from build123d import *

# Parameters (mm, degrees)
SKETCH_W            = 104.8
SKETCH_H            = 31
PAD_DEPTH           = 1.5
HOLE_D              = 3.4
HOLE_DEPTH          = 25
HOLE_CSINK_D        = 6.1
HOLE_CSINK_ANGLE    = 90
FILLET_R            = 3.5
SKETCH002_R         = 1.8
POCKET_DEPTH        = 1.501
LINEARPATTERN_COUNT = 2
LINEARPATTERN_PITCH = 81.28


with BuildPart() as part:
    # Sketch → Pad (new body)
    with BuildSketch(Plane.XZ):
        Rectangle(SKETCH_W, SKETCH_H)
    extrude(amount=PAD_DEPTH)

    # Hole
    with Locations(Plane.XZ.offset(1.5)):
        with Locations((-48.5, 11.5), (-48.5, -11.5), (48.5, -11.5), (48.5, 11.5)):
            CounterSinkHole(HOLE_D / 2, HOLE_CSINK_D / 2, depth=HOLE_DEPTH, counter_sink_angle=HOLE_CSINK_ANGLE)

    # Fillet
    fillet_edges = [part.edges().sort_by_distance(p)[0] for p in [
        (-52.4, -0.75, 15.5),
        (52.4, -0.75, 15.5),
    ]]
    fillet(fillet_edges, radius=FILLET_R)

    # Sketch002 (on Face5 of Fillet) → Pocket (cut, through all)
    with BuildSketch(Plane.XZ.offset(1.5)):
        with Locations((-40.61, 0.03)):
            Circle(SKETCH002_R)
    pocket = extrude(amount=-POCKET_DEPTH, mode=Mode.SUBTRACT)

    # LinearPattern: Pocket ×2
    with Locations(*[(i * LINEARPATTERN_PITCH, 0, 0) for i in range(1, LINEARPATTERN_COUNT)]):
        add(pocket, mode=Mode.SUBTRACT)


solid = part.part
Part model, mm, in its own coordinate system. Coordinates: 2 decimals unless noted, no trailing zeros. Order: outer loops, then holes, each group sorted by start corner. A loop starts at its lowest first (then second) coordinate and runs counter-clockwise, first axis right, second up. Notation, with made-up numbers: M 6,13.5 L 29,13.5 A15 cw 29,22.5 Z; hole C 7,85 d6. An arc over 180 degrees is marked long. Use a Markdown table: item, result.
(1) Cut at B-B on x = 40.67. Write the cut outline in (y, z), then the cut area to 3 significant figures.
A:
| item | result |
|---|---|
| outline | M -1.5,-15.5 L 0,-15.5 L 0,-1.77 L -1.5,-1.77 Z; M -1.5,1.83 L 0,1.83 L 0,15.5 L -1.5,15.5 Z |
| area | 41.1 mm^2 |
(2) Pull direction X, two halves, no side cores. Call faces 1 (the cylindrical face through (-42.41, -0.76, 0.11)), 2 (the cylindrical face through (41.501, -0.76, -1.567)), 3 (the cylindrical face through (51.4, -0.76, 14.45)), 4 (the flat face through (-1, 0, 0)): released by +X, released by -X, zero draft, split by the parting line, or undercut.
A:
| item | result |
|---|---|
| face 1 | undercut |
| face 2 | undercut |
| face 3 | released by +X |
| face 4 | zero draft |
(3) Flat gauge pins, fed straight in: pin 1 (4.5 mm diameter, centred on x = 40.67, z = 0.03, fed in from +Y); pin 2 (5.5 mm diameter, centred on x = 48.5, z = 11.5, fed in from -Y); pin 3 (2 mm diameter, centred on x = -48.5, z = -11.5, fed in from +Y). Where does each tip first touch, or does it go through?
A:
| item | result |
|---|---|
| pin 1 | stops at y = 0 |
| pin 2 | stops at y = -1.2 |
| pin 3 | passes through |
(4) Cut at C-C on y = -1.25. Write the cut outline in (x, z), then the cut area to 3 significant figures.
A:
| item | result |
|---|---|
| outline | M -52.4,-15.5 L 52.4,-15.5 L 52.4,12 A3.5 ccw 48.9,15.5 L -48.9,15.5 A3.5 ccw -52.4,12 Z; hole C -48.5,-11.5 d5.6; hole C -48.5,11.5 d5.6; hole C -40.61,0.03 d3.6; hole C 40.67,0.03 d3.6; hole C 48.5,-11.5 d5.6; hole C 48.5,11.5 d5.6 |
| area | 3,120 mm^2 |
(5) Probe L1, parallel to X at y = -0.05, z = 11.5; L2, parallel to X at y = -1.2, z = 9.5; L3, parallel to Z at x = 40.67, y = -1.1. List the from-to ranges inside material, lowest first.
A:
| item | result |
|---|---|
| L1 | x = -52.4 to -50.2, -46.8 to 46.8, 50.2 to 52.4 |
| L2 | x = -52.4 to -50.39, -46.61 to 46.61, 50.39 to 52.4 |
| L3 | z = -15.5 to -1.77, 1.83 to 15.5 |
(6) Cut at D-D on z = -11.5. Write the cut outline in (x, y), then the cut area to 3 significant figures.
A:
| item | result |
|---|---|
| outline | M -52.4,-1.5 L -51.55,-1.5 L -50.2,-0.15 L -50.2,0 L -52.4,0 Z; M -46.8,-0.15 L -45.45,-1.5 L 45.45,-1.5 L 46.8,-0.15 L 46.8,0 L -46.8,0 Z; M 50.2,-0.15 L 51.55,-1.5 L 52.4,-1.5 L 52.4,0 L 50.2,0 Z |
| area | 143 mm^2 |
(7) Cut at A-A on z = 0.03. Write the cut outline in (x, y), then the cut area to 3 significant figures.
A:
| item | result |
|---|---|
| outline | M -52.4,-1.5 L -42.41,-1.5 L -42.41,0 L -52.4,0 Z; M -38.81,-1.5 L 38.87,-1.5 L 38.87,0 L -38.81,0 Z; M 42.47,-1.5 L 52.4,-1.5 L 52.4,0 L 42.47,0 Z |
| area | 146 mm^2 |
